Autodesk Inventor part; units mm, degrees
ref_plane "YZ Plane" through (0, 0, 0) normal (1, 0, 0) x (0, 1, 0)
ref_plane "XZ Plane" through (0, 0, 0) normal (0, 1, 0) x (-1, 0, 0)
ref_plane "XY Plane" through (0, 0, 0) normal (0, 0, 1) x (1, 0, 0)
sketch "Sketch1" plane through (0, 0, 0) normal (0, 1, 0) x (-1, 0, 0)
  line L0 (0, 0) -> (-19.05, 0)
  line L1 (-19.05, 0) -> (-19.05, 133.35)
  line L2 (-19.05, 133.35) -> (0, 133.35)
  line L3 (0, 133.35) -> (0, 0)
  dimension "d0" = 19.05
  dimension "d1" = 133.35
extrude "Board" add sketch "Sketch1" along normal blind 838.2
sketch "Sketch2" plane through (19.05, 0, 133.35) normal (1, 0, 0) x (0, 0, -1)
  line L0 (0, 349.25) -> (133.35, 349.25)
  line L1 (133.35, 349.25) -> (133.35, 330.2)
  line L2 (133.35, 330.2) -> (0, 330.2)
  line L3 (0, 330.2) -> (0, 349.25)
  line L4 (0, 0) -> (133.35, 0)
  line L5 (0, 0) -> (0, 838.2)
  line L6 (133.35, 0) -> (133.35, 838.2)
  line L7 (0, 635) -> (133.35, 635)
  line L8 (133.35, 635) -> (133.35, 615.95)
  line L9 (133.35, 615.95) -> (0, 615.95)
  line L10 (0, 615.95) -> (0, 635)
  line L11 (0, 838.2) -> (133.35, 838.2)
  dimension "d4" = 19.05
  dimension "d5" = 330.2
  dimension "d9" = 19.05
  dimension "d13" = 203.2
  dimension "d14" = 266.7
extrude "Extrusion2" cut sketch "Sketch2" against normal blind 9.525 contours L0 L1 L2 L3 | L5 L7 L6 L9
sketch "Sketch3" plane through (0, 838.2, 0) normal (0, 1, 0) x (1, 0, 0)
  line L0 (0, -133.35) -> (19.05, -133.35)
  line L1 (19.05, -133.35) -> (9.525, -133.35)
  line L2 (9.525, -133.35) -> (9.525, 0)
  line L3 (9.525, 0) -> (19.05, 0)
  line L4 (19.05, 0) -> (19.05, -133.35)
  line L5 (19.05, 0) -> (0, 0)
  dimension "d15" = 9.525
extrude "Extrusion3" add sketch "Sketch3" along normal blind 9.525
sketch "Sketch4" plane through (0, 0, 0) normal (0, -1, 0) x (1, 0, 0)
  line L0 (19.05, 0) -> (9.525, 0)
  line L1 (9.525, 0) -> (9.525, 133.35)
  line L2 (9.525, 133.35) -> (19.05, 133.35)
  line L3 (19.05, 133.35) -> (19.05, 0)
  line L4 (19.05, 0) -> (19.05, 133.35)
  line L5 (0, 0) -> (19.05, 0)
  line L6 (19.05, 133.35) -> (0, 133.35)
  dimension "d18" = 9.525
extrude "Extrusion4" add sketch "Sketch4" along normal blind 9.525
sketch "Sketch5" plane through (0, 0, 0) normal (-1, 0, 0) x (0, 0, 1)
  line L0 (0, 647.7) -> (11.1125, 647.7)
  line L1 (14.2875, 644.525) -> (14.2875, 612.775)
  line L2 (11.1125, 609.6) -> (0, 609.6)
  line L3 (0, 609.6) -> (0, 647.7)
  line L4 (0, 228.6) -> (11.1125, 228.6)
  line L5 (14.2875, 225.425) -> (14.2875, 193.675)
  line L6 (11.1125, 190.5) -> (0, 190.5)
  line L7 (0, 190.5) -> (0, 228.6)
  line L8 (0, 0) -> (0, 838.2)
  line L9 (133.35, 838.2) -> (0, 838.2)
  arc A0 (11.1125, 609.6) -> (14.2875, 612.775) centre (11.1125, 612.775) ccw
  arc A1 (14.2875, 644.525) -> (11.1125, 647.7) centre (11.1125, 644.525) ccw
  arc A2 (11.1125, 190.5) -> (14.2875, 193.675) centre (11.1125, 193.675) ccw
  arc A3 (14.2875, 225.425) -> (11.1125, 228.6) centre (11.1125, 225.425) ccw
  point P0 (14.2875, 609.6)
  point P1 (14.2875, 647.7)
  point P2 (14.2875, 190.5)
  point P3 (14.2875, 228.6)
  dimension "d21" = 14.2875
  dimension "d22" = 38.1
  dimension "d23" = 14.2875
  dimension "d24" = 38.1
  dimension "d25" = 190.5
  dimension "d26" = 838.2
  dimension "d27" = 381
  dimension "d28" = 3.175
extrude "Extrusion5" cut sketch "Sketch5" against normal blind 3.175
equation "\"d9\" = d4"
equation "\"d25\" = 0.25 * d26 - 0.5 * d22"
equation "\"d27\" = 2 * d25"
properties part number "Door Side" material "Wood (Oak)"
For this review, take the finished solid that the model builds, in its own axes (mm). A direction names the side the tool comes from. Coordinates: 2 decimals unless noted, no trailing zeros. Write each loop counter-clockwise with the first axis right and the second up, starting at its lowest first coordinate (ties: lowest second). Pieces come first, ordered by that corner, then holes. Notation, with made-up numbers: (-8.5, -4.75) -> (43.5, -4.75) arc R19 cw to (43.5, 5.25) -> close; hole circle Ø4 at (-22, -1). An arc over 180 degrees is marked (long way). Write each question's results on one line, items separated by ' | '. Start each with the question number.
1) Insertion check: pin 1 (2.5 mm diameter, centred on x = 2.5, z = 3.5, fed in from +Y); pin 2 (1.6 mm diameter, centred on x = 1.5, z = 4, fed in from -Y); pin 3 (5.5 mm diameter, centred on y = 630, z = 82, fed in from +X) (3 decimals). Each pin has a flat end and moves straight along its axis. Give the tip position at first contact, or say it passes through.
2) Wall thickness on L1, parallel to Y at x = 12.5, z = 122.5 (3 decimals); L2, parallel to Y at x = 7, z = 43: over which ranges is each line inside the solid? List them lowest first. Write a range as [from, to].
3) The part is to be moulded in two halves that separate along Y. For faces 4 (the face through (9, 425, 133.35)), 5 (the face through (9.525, 340, 68)), say which applies: +Y half, -Y half, draft (parallel to the pull), parting line (faces both ways), or undercut.
4) For faces 1 (the face through (9.525, 626, 68)), 2 (the face through (3.175, 210, 7)), 3 (the face through (0, 413, 68)), list the 3-axis set-ups (+Z, -Z, +X, -X, +Y, -Y) from which the entire face can be reached by the end or side of a thin tool; tool diameter is ignored.
5) Consider section A-A (x = 14.25). Write out the cut boundary in (y, z) (3 decimals), plus the area to 3 significant figures.
6) Consider section B-B (z = 71.5). Write out the cut boundary in (x, y) (3 decimals).
Geometry says:
1) pin 1: y = 838.2 | pin 2: y = 0 | pin 3: x = 9.525
2) L1: [-9.525, 330.2], [349.25, 615.95], [635, 847.725] | L2: [0, 838.2]
3) face 4: draft | face 5: undercut
4) face 1: +Z, -Z, +X | face 2: -Z, -X | face 3: +Z, -Z, -X, +Y, -Y
5) outline: (-9.525, 0) -> (330.2, 0) -> (330.2, 133.35) -> (-9.525, 133.35) -> close; (349.25, 0) -> (615.95, 0) -> (615.95, 133.35) -> (349.25, 133.35) -> close; (635, 0) -> (847.725, 0) -> (847.725, 133.35) -> (635, 133.35) -> close | area: 109,000 mm^2
6) outline: (0, 0) -> (9.525, 0) -> (9.525, -9.525) -> (19.05, -9.525) -> (19.05, 330.2) -> (9.525, 330.2) -> (9.525, 349.25) -> (19.05, 349.25) -> (19.05, 615.95) -> (9.525, 615.95) -> (9.525, 635) -> (19.05, 635) -> (19.05, 847.725) -> (9.525, 847.725) -> (9.525, 838.2) -> (0, 838.2) -> close
